The listing builds one solid part. Answer for the finished solid, in the listing's coordinates (mm). Face numbers are marked on the shaded views. A direction names the side the tool comes from. Give positions to 0.01 mm unless a question says otherwise; leave off trailing zeros. Write each loop counter-clockwise with the first axis right and the second up, starting at its lowest first coordinate (ties: lowest second). Pieces come first, ordered by that corner, then holes. Notation, with made-up numbers: M -18,-16 L 0,-16 A16 ccw 0,1 Z; hole C 74,9.25 d5. An arc over 180 degrees is marked long. Answer as a JSON object with one key per item and string values.
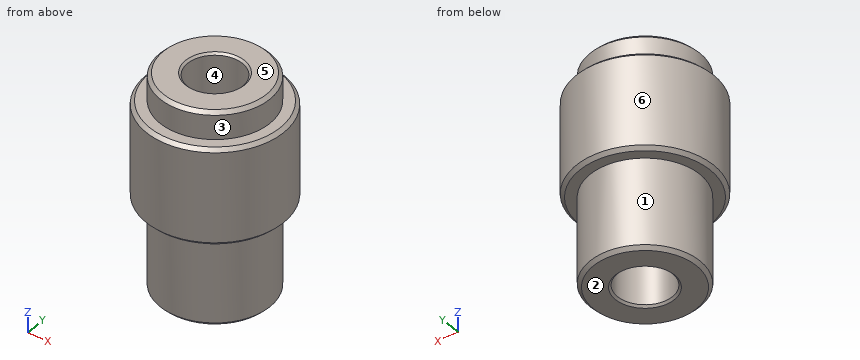
```python
from build123d import *

# Parameters (mm, degrees)
CHAMFER_1_SIZE      = 0.25
SKETCH_2_R          = 2
CUT_EXTRUDE_1_DEPTH = 18.036725037
CHAMFER_2_SIZE      = 0.15


with BuildPart() as part:
    # ｽｹｯﾁ1 → 回転1 (revolve)
    with BuildSketch(Plane(origin=(0, 0, 0), x_dir=(0, 0, -1), z_dir=(1, 0, 0)), mode=Mode.PRIVATE) as revolve_1_sk:
        Polygon((0, 0), (0, 4), (2, 4), (2, 5), (9, 5), (9, 4), (15.5, 4), (15.5, 0), align=None)
    revolve(revolve_1_sk.sketch.rotate(Axis((0, 0, -15.5), (0, 0, 1)), 90), axis=Axis((0, 0, -15.5), (0, 0, 1)))

    # 面取り1
    chamfer_1_edges = [part.edges().sort_by_distance(p)[0] for p in [
        (4, 0, -15.5),
        (5, 0, -9),
        (5, 0, -2),
        (4, 0, 0),
    ]]
    chamfer(chamfer_1_edges, length=CHAMFER_1_SIZE)

    # ｽｹｯﾁ2 → ｶｯﾄ - 押し出し1 (cut, through all)
    with BuildSketch(Plane.XY):
        Circle(SKETCH_2_R)
    extrude(amount=-CUT_EXTRUDE_1_DEPTH, mode=Mode.SUBTRACT)

    # 面取り2
    chamfer_2_edges = [part.edges().sort_by_distance(p)[0] for p in [
        (-2, 0, -15.5),
        (-2, 0, 0),
    ]]
    chamfer(chamfer_2_edges, length=CHAMFER_2_SIZE)


solid = part.part
```
1. A cutting plane is placed at C-C, the plane z = -12.75. Give the vertices of the cut face in (x, y), plus the area to 3 significant figures.
Verdict:
{"outline": "C 0,0 d8; hole C 0,0 d4", "area": "37.7 mm2"}
2. Flat-ended cylindrical pins translate along their axes: pin 1 (5 mm diameter, centred on x = 2, y = 1, fed in from +Z); pin 2 (5 mm diameter, centred on y = -3, z = -5, fed in from +X); pin 3 (3 mm diameter, centred on x = -2.5, z = -2, fed in from -Y); pin 4 (1.5 mm diameter, centred on y = -3.5, z = -3, fed in from -X). Find the tip coordinate at first contact, or state that the pin passes through.
Verdict:
{"pin 1": "stops at z = 0", "pin 2": "stops at x = 4.97", "pin 3": "stops at y = -4.89", "pin 4": "stops at x = -4.18"}
3. The mould has two halves that part along X. Classify the marked faces 4, 5 and 6: released by +X, released by -X, zero draft, split by the parting line, or undercut.
Verdict:
{"face 4": "undercut", "face 5": "zero draft", "face 6": "split by the parting line"}
4. A cutting plane is placed at A-A, the plane x = 0. Give the vertices of the cut face in (y, z).
Verdict:
{"outline": "M -5,-8.75 L -4.75,-9 L -4,-9 L -4,-15.25 L -3.75,-15.5 L -2.15,-15.5 L -2,-15.35 L -2,-0.15 L -2.15,0 L -3.75,0 L -4,-0.25 L -4,-2 L -4.75,-2 L -5,-2.25 Z; M 2,-15.35 L 2.15,-15.5 L 3.75,-15.5 L 4,-15.25 L 4,-9 L 4.75,-9 L 5,-8.75 L 5,-2.25 L 4.75,-2 L 4,-2 L 4,-0.25 L 3.75,0 L 2.15,0 L 2,-0.15 Z"}
5. For the marked faces 1, 2 and 3, determine the directions among +Z, -Z, +X, -X, +Y, -Y from which every point of the face is accessible in a straight line to the end or side of a thin tool.
Verdict:
{"face 1": "-Z", "face 2": "-Z, +X, -X, +Y, -Y", "face 3": "+Z"}
6. Consider line 1 along Y through (x, z) = (0, -4.75); line 2 along Y through (x, z) = (0, -12.25); line 3 along Z through (x, y) = (0.5, 4.25). Determine where each line is inside the solid, lowest interval first.
Verdict:
{"line 1": "y = -5 to -2, 2 to 5", "line 2": "y = -4 to -2, 2 to 4", "line 3": "z = -9 to -2"}
7. A cutting plane is placed at D-D, the plane z = -3. Give the vertices of the cut face in (x, y), plus the area to 3 significant figures.
Verdict:
{"outline": "C 0,0 d10; hole C 0,0 d4", "area": "66.0 mm2"}
